Source: three-view drawing plus pictorial views. Frame: mm from the lowest corner of the part. A direction names the side the tool comes from. Give positions to 0.01 mm unless a question says otherwise; leave off trailing zeros. Write each loop counter-clockwise with the first axis right and the second up, starting at its lowest first coordinate (ties: lowest second). Pieces come first, ordered by that corner, then holes.
Q1. Reachability of the marked faces 4, 5 and 6 from +Z, -Z, +X, -X, +Y, -Y: full face, straight path, thin tool, end or side. Return the list, or none.
Q2. Cut plane A-A on x = 31.1. Return the cut outline in (y, z) (3 decimals), plus the area to 3 significant figures.
Q3. Line query: L1, parallel to Y at x = 10, z = 1.3; L2, parallel to X at y = 5.5, z = 1.05; L3, parallel to X at y = 5.75, z = 1.9. Output: solid intervals per line, ascending.
Q4. Pin query (flat end, axial travel): pin 1 (1.6 mm diameter, centred on x = 38, z = 1, fed in from -Y); pin 2 (1.6 mm diameter, centred on x = 39, z = 2, fed in from +Y); pin 3 (1.6 mm diameter, centred on y = 2.5, z = 1, fed in from -X). Return the tip coordinate at first contact, or that it passes through.
Q5. Cut plane B-B on y = 5. Return the cut outline in (x, z) (3 decimals), plus the area to 3 significant figures.
Q6. Cut plane C-C on z = 1.8. Return the cut outline in (x, y).
Q7. Cut plane D-D on y = 7.75. Return the cut outline in (x, z) (3 decimals), plus the area to 3 significant figures.
Q8. Draft query along Y for the marked faces 1, 2 and 3. Return one class per face: pulls with the +Y half, pulls with the -Y half, needs draft (parallel to the pull), parting line crosses it, or undercut.
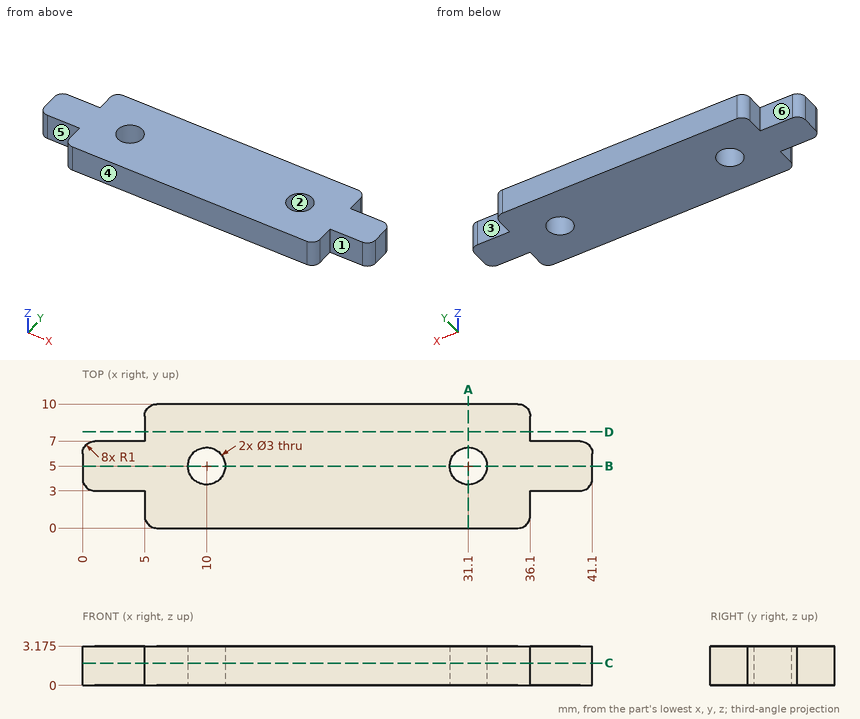
Data:
1. face 4: +Z, -Z, +X, -X, -Y
1. face 5: +Z, -Z, -X, -Y
1. face 6: +Z, -Z, -X, +Y
2. outline: (0, 0) - (3.5, 0) - (3.5, 3.175) - (0, 3.175) - close; (6.5, 0) - (10, 0) - (10, 3.175) - (6.5, 3.175) - close
2. area: 22.2 mm2
3. L1: y = 0 to 3.5, 6.5 to 10
3. L2: x = 0 to 8.59, 11.41 to 29.69, 32.51 to 41.1
3. L3: x = 0 to 8.7, 11.3 to 29.8, 32.4 to 41.1
4. pin 1: stops at y = 3
4. pin 2: stops at y = 7
4. pin 3: stops at x = 0.29
5. outline: (0, 0) - (8.5, 0) - (8.5, 3.175) - (0, 3.175) - close; (11.5, 0) - (29.6, 0) - (29.6, 3.175) - (11.5, 3.175) - close; (32.6, 0) - (41.1, 0) - (41.1, 3.175) - (32.6, 3.175) - close
5. area: 111 mm2
6. outline: (0, 4) arc R1 ccw to (1, 3) - (5, 3) - (5, 1) arc R1 ccw to (6, 0) - (35.1, 0) arc R1 ccw to (36.1, 1) - (36.1, 3) - (40.1, 3) arc R1 ccw to (41.1, 4) - (41.1, 6) arc R1 ccw to (40.1, 7) - (36.1, 7) - (36.1, 9) arc R1 ccw to (35.1, 10) - (6, 10) arc R1 ccw to (5, 9) - (5, 7) - (1, 7) arc R1 ccw to (0, 6) - close; hole circle Ø3 at (10, 5); hole circle Ø3 at (31.1, 5)
7. outline: (5, 0) - (36.1, 0) - (36.1, 3.175) - (5, 3.175) - close
7. area: 98.7 mm2
8. face 1: pulls with the -Y half
8. face 2: undercut
8. face 3: pulls with the +Y half
